from build123d import *

# Parameters (mm, degrees)
SKETCH1_W               = 124.5
SKETCH1_H               = 85
BOSS_EXTRUDE1_DEPTH     = 4.5
SKETCH2_W               = 85
SKETCH2_H               = 4.5
BOSS_EXTRUDE2_DEPTH     = 95
SKETCH3_W               = 80.5
SKETCH3_H               = 2
BOSS_EXTRUDE3_DEPTH     = 90.5
SKETCH4_W               = 8
SKETCH4_H               = 2
BOSS_EXTRUDE4_DEPTH     = 8
SKETCH5_W               = 8
SKETCH5_H               = 2
BOSS_EXTRUDE5_DEPTH     = 8
CUT_EXTRUDE1_DEPTH      = 183.576696213
CUT_EXTRUDE1_DEPTH_BACK = 183.576696213
SKETCH6_R               = 1.7
FILLET1_R               = 2


with BuildPart() as part:
    # Sketch1 → Boss-Extrude1 (new body)
    with BuildSketch(Plane(origin=(0, 0, 0), x_dir=(0, 1, 0), z_dir=(0, 0, 1))):
        with Locations((62.25, 42.5)):
            Rectangle(SKETCH1_W, SKETCH1_H)
    extrude(amount=BOSS_EXTRUDE1_DEPTH)

    # Sketch2 → Boss-Extrude2 (add)
    with BuildSketch(Plane(origin=(0, 0, 0), x_dir=(1, 0, 0), z_dir=(0, 0, -1))):
        with Locations((-42.5, -2.25)):
            Rectangle(SKETCH2_W, SKETCH2_H)
    extrude(amount=BOSS_EXTRUDE2_DEPTH)

    # Sketch3 → Boss-Extrude3 (add)
    with BuildSketch(Plane(origin=(0, 0, 0), x_dir=(1, 0, 0), z_dir=(0, 0, -1))):
        with Locations((-42.5, -5.5)):
            Rectangle(SKETCH3_W, SKETCH3_H)
    extrude(amount=BOSS_EXTRUDE3_DEPTH)

    # Sketch4 → Boss-Extrude4 (add)
    with BuildSketch(Plane.XY.offset(4.5)):
        with Locations((-76.5, 123.5)):
            Rectangle(SKETCH4_W, SKETCH4_H)
        with Locations((-8.5, 123.5)):
            Rectangle(SKETCH4_W, SKETCH4_H)
    extrude(amount=BOSS_EXTRUDE4_DEPTH)

    # Sketch5 → Boss-Extrude5 (add)
    with BuildSketch(Plane(origin=(0, 0, -95), x_dir=(1, 0, 0), z_dir=(0, 0, -1))):
        with Locations((-76.5, -3.5)):
            Rectangle(SKETCH5_W, SKETCH5_H)
        with Locations((-8.5, -3.5)):
            Rectangle(SKETCH5_W, SKETCH5_H)
    extrude(amount=BOSS_EXTRUDE5_DEPTH)

    # Sketch6 → Cut-Extrude1 (cut, two sides: drawn at the far end of the back side and taken through both)
    with BuildSketch(Plane(origin=(0, 124.5, 0), x_dir=(-1, 0, 0), z_dir=(0, 1, 0)).offset(-CUT_EXTRUDE1_DEPTH_BACK)):
        with Locations(Location((8.5, 8.5, 0), (0, 0, 90))):
            Circle(SKETCH6_R)
        with Locations(Location((76.5, 8.5, 0), (0, 0, 90))):
            Circle(SKETCH6_R)
        with Locations(Location((76.5, -99, 0), (0, 0, 90))):
            Circle(SKETCH6_R)
        with Locations(Location((8.5, -99, 0), (0, 0, 90))):
            Circle(SKETCH6_R)
    extrude(amount=CUT_EXTRUDE1_DEPTH + CUT_EXTRUDE1_DEPTH_BACK, mode=Mode.SUBTRACT)

    # Fillet1
    fillet1_edges = [part.edges().sort_by_distance(p)[0] for p in [
        (-80.5, 123.5, 4.5),
        (-72.5, 123.5, 4.5),
        (-80.5, 123.5, 12.5),
        (-72.5, 123.5, 12.5),
        (-4.5, 123.5, 4.5),
        (-12.5, 123.5, 4.5),
        (-4.5, 123.5, 12.5),
        (-12.5, 123.5, 12.5),
        (-80.5, 3.5, -95),
        (-72.5, 3.5, -95),
        (-80.5, 3.5, -103),
        (-72.5, 3.5, -103),
        (-4.5, 3.5, -95),
        (-12.5, 3.5, -95),
        (-4.5, 3.5, -103),
        (-12.5, 3.5, -103),
    ]]
    fillet(fillet1_edges, radius=FILLET1_R)


solid = part.part
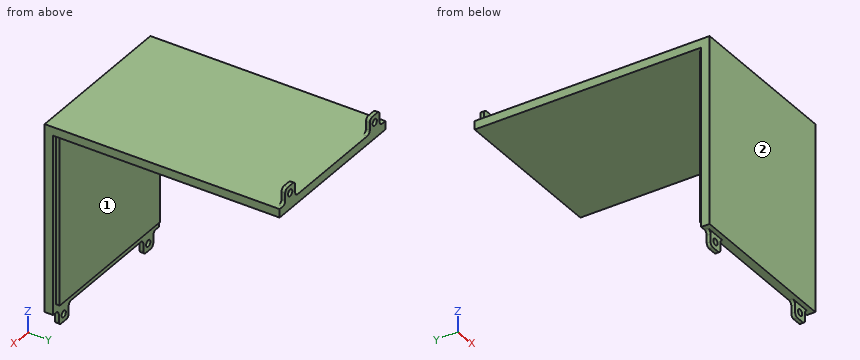
CAD build for the part. Positions are in the model's coordinates, mm. Face numbers are marked on the shaded views. A direction names the side the tool comes from. Coordinates: 2 decimals unless noted, no trailing zeros. Write each loop counter-clockwise with the first axis right and the second up, starting at its lowest first coordinate (ties: lowest second). Pieces come first, ordered by that corner, then holes. Notation, with made-up numbers: M 38.5,86.5 L 46.5,86.5 A24 cw 46.5,107.5 Z; hole C -18,37.5 d10. An arc over 180 degrees is marked long. Answer as a JSON object with one key per item and string values. Group by question number.
1) Saw through at B-B (x = -8.5). Write the cut outline in (y, z), plus the area to 3 significant figures.
2) Saw through at D-D (z = -29). Write the cut outline in (x, y).
3) Saw through at C-C (x = -55.5). Write the cut outline in (y, z).
4) Pin check, flat tips, straight feed: pin 1 Ø2 at (x, z) = (-14.5, -17.5) entering from -Y; pin 2 Ø1.6 at (y, z) = (3, -98.5) entering from -X; pin 3 Ø4.5 at (x, z) = (-8.5, -99) entering from -Y; pin 4 Ø1.6 at (y, z) = (123.5, 8.5) entering from +X. Stop position of each tip, or through.
5) Wall check: line 1 (X direction, y = 3, z = -99); line 2 (X direction, y = 123, z = 8); line 3 (Z direction, x = -8.5, y = 123.1). Give the ranges that are in metal, low to high. Write a range as from..to.
6) Saw through at A-A (z = 8.5). Write the cut outline in (x, y), plus the area to 3 significant figures.
7) Tool access for the marked faces 1 and 2: list every direction of +Z, -Z, +X, -X, +Y, -Y with a clear straight run to the whole face (end or side of a thin tool).
Values follow:
{
 "1": {"outline": "M 0,-95 L 2.5,-95 L 2.5,-97.3 L 4.5,-97.3 L 4.5,-90.5 L 6.5,-90.5 L 6.5,0 L 124.5,0 L 124.5,6.8 L 122.5,6.8 L 122.5,4.5 L 0,4.5 Z; M 2.5,-103 L 4.5,-103 L 4.5,-100.7 L 2.5,-100.7 Z; M 122.5,10.2 L 124.5,10.2 L 124.5,12.5 L 122.5,12.5 Z", "area": "1,190 mm2"},
 "2": {"outline": "M -85,0 L 0,0 L 0,4.5 L -2.25,4.5 L -2.25,6.5 L -82.75,6.5 L -82.75,4.5 L -85,4.5 Z"},
 "3": {"outline": "M 0,-95 L 4.5,-95 L 4.5,-90.5 L 6.5,-90.5 L 6.5,0 L 124.5,0 L 124.5,4.5 L 0,4.5 Z"},
 "4": {"pin 1": "stops at y = 0", "pin 2": "stops at x = -80.5", "pin 3": "stops at y = 2.5", "pin 4": "stops at x = -4.5"},
 "5": {"line 1": "x = -80.5..-78.2, -74.8..-72.5, -12.5..-10.2, -6.8..-4.5", "line 2": "x = -80.5..-78.12, -74.88..-72.5, -12.5..-10.12, -6.88..-4.5", "line 3": "z = 0..6.8, 10.2..12.5"},
 "6": {"outline": "M -80.5,122.5 L -78.2,122.5 L -78.2,124.5 L -80.5,124.5 Z; M -74.8,122.5 L -72.5,122.5 L -72.5,124.5 L -74.8,124.5 Z; M -12.5,122.5 L -10.2,122.5 L -10.2,124.5 L -12.5,124.5 Z; M -6.8,122.5 L -4.5,122.5 L -4.5,124.5 L -6.8,124.5 Z", "area": "18.4 mm2"},
 "7": {"face 1": "-Z, +X, -X, +Y", "face 2": "+Z, -Z, +X, -X, -Y"}
}
